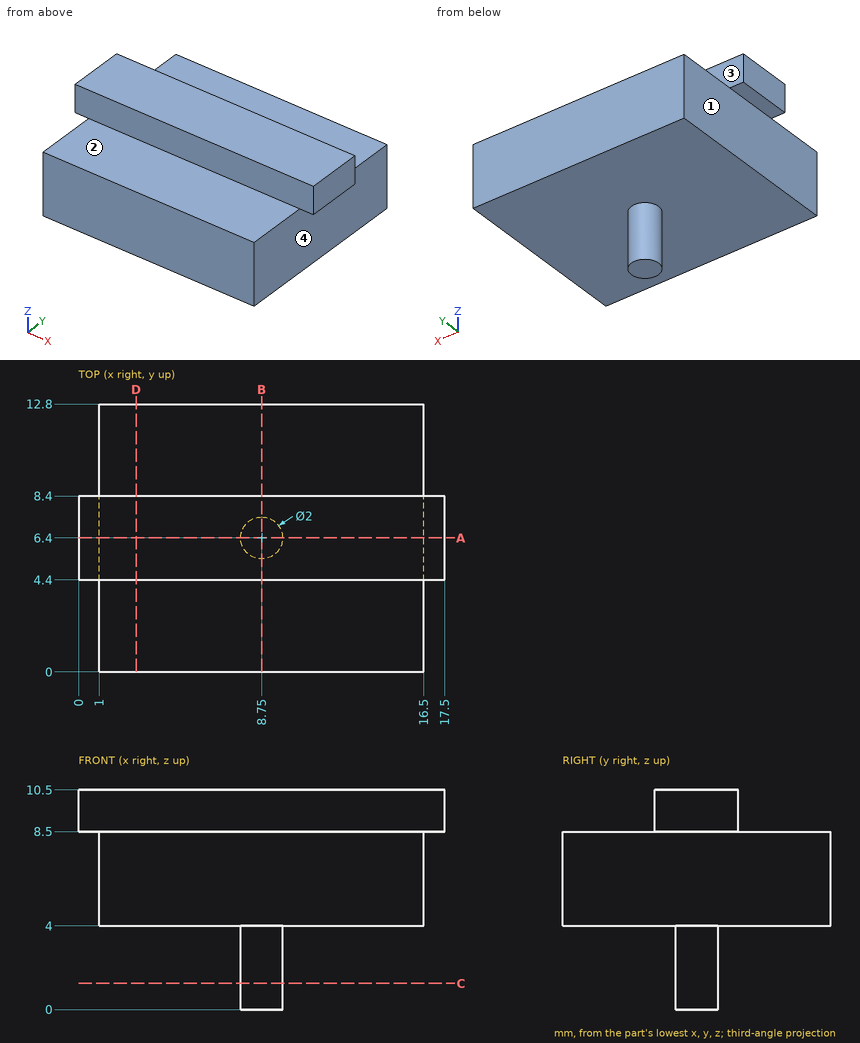
Geometry: see drawing. Coordinates: mm, zero at the bounding-box minimum. A direction names the side the tool comes from. Round coordinates to 2 decimals unless told otherwise and drop trailing zeros. Order: outer loops, then holes, each group sorted by start corner. A loop starts at its lowest first (then second) coordinate and runs counter-clockwise, first axis right, second up. Notation, with made-up numbers: (26, 72) - (31, 72) arc R15 cw to (31, 92) - close; hole circle Ø10 at (-23, -36). An arc over 180 degrees is marked (long way). Use a Markdown table: item, result. Add a question column.
1. Set-up query: the marked faces 1, 2, 3 and 4. Return all of +Z, -Z, +X, -X, +Y, -Y with unobstructed straight access to the full face (end or side cutting, diameter ignored); none if empty.
2. Line query: probe 1 along Y at (x, z) = (14.75, 9.25); probe 2 along Z at (x, y) = (4, 6); probe 3 along Z at (x, y) = (10.5, 9.25). Output: solid intervals per line, ascending.
3. Section query B-B (x = 8.75). Return the cut outline in (y, z), then the cut area to 3 significant figures.
4. First-contact query: pin 1 (1.6 mm diameter, centred on x = 13, z = 9.5, fed in from +Y); pin 2 (0.5 mm diameter, centred on x = 0.5, y = 7, fed in from -Z); pin 3 (2 mm diameter, centred on x = 8.5, y = 11, fed in from +Z); pin 4 (5 mm diameter, centred on x = 9.5, z = 5.5, fed in from -Y). Flat tips, straight axial feed; report the tip coordinate or a pass-through.
5. Section query A-A (y = 6.4). Return the cut outline in (x, z).
6. Section query C-C (z = 1.25). Return the cut outline in (x, y).
7. Section query D-D (x = 2.75). Return the cut outline in (y, z).
Derived:
| question | item | result |
|---|---|---|
| 1 | face 1 | -Z, -X, +Y, -Y |
| 1 | face 2 | +Z, +X, -X, -Y |
| 1 | face 3 | +Z, +X, -X, +Y |
| 1 | face 4 | -Z, +X, +Y, -Y |
| 2 | probe 1 | 4.4 to 8.4 |
| 2 | probe 2 | 4 to 10.5 |
| 2 | probe 3 | 4 to 8.5 |
| 3 | outline | (0, 4) - (5.4, 4) - (5.4, 0) - (7.4, 0) - (7.4, 4) - (12.8, 4) - (12.8, 8.5) - (8.4, 8.5) - (8.4, 10.5) - (4.4, 10.5) - (4.4, 8.5) - (0, 8.5) - close |
| 3 | area | 73.6 mm2 |
| 4 | pin 1 | y = 8.4 |
| 4 | pin 2 | z = 8.5 |
| 4 | pin 3 | z = 8.5 |
| 4 | pin 4 | y = 0 |
| 5 | outline | (0, 8.5) - (1, 8.5) - (1, 4) - (7.75, 4) - (7.75, 0) - (9.75, 0) - (9.75, 4) - (16.5, 4) - (16.5, 8.5) - (17.5, 8.5) - (17.5, 10.5) - (0, 10.5) - close |
| 6 | outline | circle Ø2 at (8.75, 6.4) |
| 7 | outline | (0, 4) - (12.8, 4) - (12.8, 8.5) - (8.4, 8.5) - (8.4, 10.5) - (4.4, 10.5) - (4.4, 8.5) - (0, 8.5) - close |
